Geometry: final body of the model. Coordinates: model frame, mm. A direction names the side the tool comes from. Give positions to 0.01 mm unless a question says otherwise; leave off trailing zeros. Loops run counter-clockwise (first coordinate to the right, second up) from the corner with the lowest first, then second, coordinate; pieces in that order, holes last.
1. First-contact query: P1, Ø21, axis at x = -13, y = 27, coming from the +Z side; P2, Ø22, axis at x = 6.5, z = 44.5, coming from the -Y side. Flat tips, straight axial feed; report the tip coordinate or a pass-through.
2. Access query for faces 4 (the face through (9, -7.5, 37)), 5 (the face through (47, -15, 29)), 6 (the face through (5, 28, 17.964)). Directions: +Z, -Z, +X, -X, +Y, -Y. A direction counts if a zero-diameter tool reaches every point of the face in a straight line with its end or side. Return the directions, or none.
3. Material intervals for line 1 along Y through (x, z) = (50, 42); line 2 along X through (y, z) = (32, 5.5); line 3 along Z through (x, y) = (-33.5, -9), sorted ascending.
4. Section A-A, the plane z = -2.5. Output: boundary loops of the cut face in (x, y), then the cut area to 3 significant figures.
5. Section B-B, the plane y = 26.5. Output: boundary loops of the cut face in (x, z), then the cut area to 3 significant figures.
6. Draft query along Z for faces 1 (the face through (54.6, -0.21, 28.85)), 2 (the face through (5, -29, 17.964)), 3 (the face through (47, 15, 29)). Return one class per face: +Z half, -Z half, draft (parallel to the pull), parting line (faces both ways), or undercut.
from build123d import *

# Parameters (mm, degrees)
F1_DEPTH = 50
F2_DEPTH = 15
F3_DEPTH = 7.5


with BuildPart() as f1:
    # F0 (on Front) → F1 (new body, symmetric)
    with BuildSketch(Plane.XZ):
        Polygon((17.809639, 17.96415), (-45.859891, 17.96415), (-45.859891, -32.03585), (54.140109, -32.03585), (54.140109, 17.96415), align=None)
    extrude(amount=F1_DEPTH, both=True)

    # F0 (on Front) → F2 (join, symmetric)
    with BuildSketch(Plane.XZ):
        with BuildLine():
            ThreePointArc((65.37061, 46.769912), (37.400469, 39.284538), (17.809639, 17.96415))
            Line((17.809639, 17.96415), (54.140109, 17.96415))
            ThreePointArc((54.140109, 17.96415), (54.702773, 28.977132), (65.37061, 31.769912))
            Line((65.37061, 31.769912), (65.37061, 46.769912))
        make_face()
    extrude(amount=F2_DEPTH, both=True)

    # F0 (on Front) → F3 (join, symmetric)
    with BuildSketch(Plane.XZ):
        with BuildLine():
            add(Edge.make_bspline(
                [(65.37061, 61.769912), (17.809639, 43.326717), (-11.461159, 66.434294), (-45.859891, 17.96415)],
                knots=[0, 0, 0, 0, 119.545679, 119.545679, 119.545679, 119.545679], degree=3))
            Line((-45.859891, 17.96415), (17.809639, 17.96415))
            ThreePointArc((17.809639, 17.96415), (37.400469, 39.284538), (65.37061, 46.769912))
            Line((65.37061, 46.769912), (65.37061, 61.769912))
        make_face()
    extrude(amount=F3_DEPTH, both=True)


solid = f1.part
Answers below:
1. P1: stops at z = 17.96
1. P2: stops at y = -7.5
2. face 4: +Z, -X, -Y
2. face 5: +Z, +X, -X, -Y
2. face 6: +Z, -X, +Y
3. line 1: y = -15 to 15
3. line 2: x = -45.86 to 54.14
3. line 3: z = -32.04 to 17.96
4. outline: (-45.86, -50) - (54.14, -50) - (54.14, 50) - (-45.86, 50) - close
4. area: 10,000 mm2
5. outline: (-45.86, -32.04) - (54.14, -32.04) - (54.14, 17.96) - (-45.86, 17.96) - close
5. area: 5,000 mm2
6. face 1: undercut
6. face 2: +Z half
6. face 3: draft
